Geometry check sheet. Reference: the model listing, model coordinates, mm. Face numbers are marked on the shaded views. A direction names the side the tool comes from. Coordinates: 2 decimals unless noted, no trailing zeros. Order: outer loops, then holes, each group sorted by start corner. A loop starts at its lowest first (then second) coordinate and runs counter-clockwise, first axis right, second up. Notation, with made-up numbers: (80.25, 29) - (84.25, 29) arc R22 cw to (84.25, 43) - close; hole circle Ø4 at (-5, -10.75). An arc over 180 degrees is marked (long way). Use CSV: the item, a comma, the result in double quotes. Start each with the question number.
1) Depth check by flat-ended pin: P1, Ø2, axis at x = -21, z = 3, coming from the -Y side; P2, Ø1, axis at y = 8, z = 5.5, coming from the +X side; P3, Ø2.5, axis at x = -13.5, y = 6.5, coming from the -Z side; P4, Ø5, axis at y = 4.5, z = -6.5, coming from the +X side. Enter the tip coordinate at first touch or a pass-through.
2) Tool access check on the marked faces 5, 6 and 7. Record the directions out of +Z, -Z, +X, -X, +Y, -Y that give a thin tool (end or side, any length) a straight path to the whole face; none if there is none.
3) Sectioned sample at B-B, the plane z = 0. Record the cut outline in (x, y).
4) Sectioned sample at D-D, the plane x = 5.5. Record the cut outline in (y, z), and give its area (3 significant figures).
5) Thickness scan on probe 1 along X at (y, z) = (6.25, 0); probe 2 along Z at (x, y) = (-12, 9.25); probe 3 along Z at (x, y) = (-2.5, 3). Record the ranges inside material, lowest first. Write a range as [from, to].
6) Sectioned sample at C-C, the plane x = -4.5. Record the cut outline in (y, z).
7) Sectioned sample at A-A, the plane y = 6.25. Record the cut outline in (x, z).
8) Draft check along X on the marked faces 1, 2, 3 and 4. Enter one of: released by +X, released by -X, zero draft, split by the parting line, or undercut.
from build123d import *

# Parameters (mm, degrees)
SKETCH_1_R      = 5
EXTRUDE_1_DEPTH = 10


with BuildPart() as part:
    # 草圖1 → 填料-伸長1 (new body)
    with BuildSketch(Plane(origin=(0, 0, 0), x_dir=(1, 0, 0), z_dir=(0, 1, 0))):
        with BuildLine():
            ThreePointArc((0, -10), (10, 0), (0, 10))
            Line((0, 10), (-10, 10))
            Line((-10, 10), (-10, 5))
            Line((-10, 5), (-15, 5))
            Line((-15, 5), (-15, 10))
            Line((-15, 10), (-25, 10))
            Line((-25, 10), (-25, -10))
            Line((-25, -10), (-15, -10))
            Line((-15, -10), (-15, -5))
            Line((-15, -5), (-10, -5))
            Line((-10, -5), (-10, -10))
            Line((-10, -10), (0, -10))
        make_face()
        Circle(SKETCH_1_R, mode=Mode.SUBTRACT)
    extrude(amount=EXTRUDE_1_DEPTH)


solid = part.part
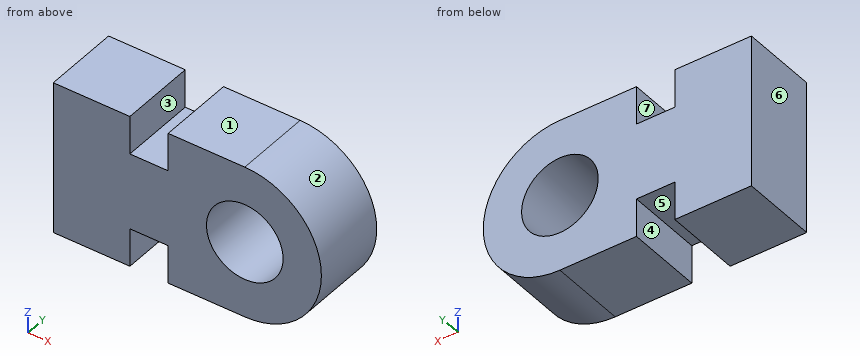
Evaluation:
1,P1,"y = 0"
1,P2,"x = 8.66"
1,P3,"z = -5"
1,P4,"x = 9.17"
2,face 5,"-Z, +Y, -Y"
2,face 6,"+Z, -Z, -X, +Y, -Y"
2,face 7,"+Z, +Y, -Y"
3,outline,"(-25, 0) - (-5, 0) - (-5, 10) - (-25, 10) - close; (5, 0) - (10, 0) - (10, 10) - (5, 10) - close"
4,outline,"(0, -8.35) - (10, -8.35) - (10, 8.35) - (0, 8.35) - close"
4,area,"167 mm²"
5,probe 1,"[-25, -5], [5, 10]"
5,probe 2,"[-5, 5]"
5,probe 3,"[-10, -4.33], [4.33, 10]"
6,outline,"(0, -10) - (10, -10) - (10, -2.18) - (0, -2.18) - close; (0, 2.18) - (10, 2.18) - (10, 10) - (0, 10) - close"
7,outline,"(-25, -10) - (-15, -10) - (-15, -5) - (-10, -5) - (-10, -10) - (0, -10) arc R10 ccw to (0, 10) - (-10, 10) - (-10, 5) - (-15, 5) - (-15, 10) - (-25, 10) - close; hole circle Ø10 at (0, 0)"
8,face 1,"zero draft"
8,face 2,"released by +X"
8,face 3,"undercut"
8,face 4,"undercut"
